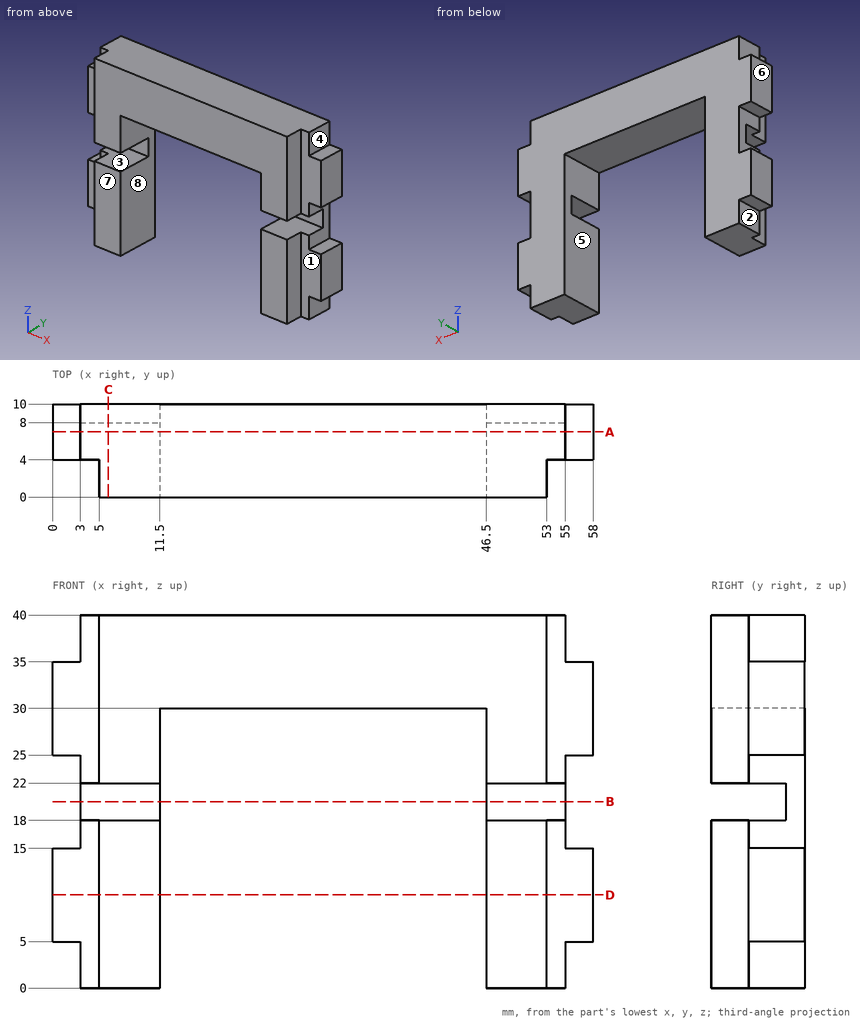
Print and shaded views of the part. All mm, measured from the part's lowest x, y and z. A direction names the side the tool comes from. Round coordinates to 2 decimals unless told otherwise and drop trailing zeros. Loops run counter-clockwise (first coordinate to the right, second up) from the corner with the lowest first, then second, coordinate; pieces in that order, holes last. Notation, with made-up numbers: M 68,1.25 L 120,1.25 A6 cw 120,11.25 Z; hole C 28,74.5 d2. An arc over 180 degrees is marked long. One line per question, with ' | ' between items.
1) Band-saw the part on C-C (x = 6). Give the cut face in (y, z), then the cut area to 3 significant figures.
Solved:
outline: M 0,0 L 10,0 L 10,40 L 0,40 L 0,22 L 8,22 L 8,18 L 0,18 Z | area: 368 mm²
2) Band-saw the part on D-D (z = 10). Give the cut face in (x, y), then the cut area to 3 significant figures.
Solved:
outline: M 0,4 L 5,4 L 5,0 L 11.5,0 L 11.5,10 L 0,10 Z; M 46.5,0 L 53,0 L 53,4 L 58,4 L 58,10 L 46.5,10 Z | area: 190 mm²
3) Drill centre lines: line 1 along Z through (x, y) = (50.5, 2.75); line 2 along X through (y, z) = (8.75, 26); line 3 along X through (y, z) = (2.75, 14). Where is each one in solid material? Low to high.
Solved:
line 1: z = 0 to 18, 22 to 40 | line 2: x = 0 to 11.5, 46.5 to 58 | line 3: x = 5 to 11.5, 46.5 to 53
4) Band-saw the part on B-B (z = 20). Give the cut face in (x, y), then the cut area to 3 significant figures.
Solved:
outline: M 3,8 L 11.5,8 L 11.5,10 L 3,10 Z; M 46.5,8 L 55,8 L 55,10 L 46.5,10 Z | area: 34.0 mm²
5) 3-axis set-ups, long thin cutter, end or side, ignore diameter. For the marked faces 1, 2, 3, 4 and 5: which of +Z, -Z, +X, -X, +Y, -Y reach the whole face in a straight line?
Solved:
face 1: +Z, -Z, +X, -Y | face 2: -Z, -X, +Y, -Y | face 3: +X, -X, -Y | face 4: +Z, +X, +Y, -Y | face 5: -Z, +Y, -Y
6) Flat gauge pins, fed straight in: pin 1 (3 mm diameter, centred on x = 31, y = 2.5, fed in from -Z); pin 2 (1.5 mm diameter, centred on y = 8.5, z = 2.5, fed in from +X); pin 3 (2.5 mm diameter, centred on x = 2, y = 6, fed in from -Z); pin 4 (0.9 mm diameter, centred on x = 1, y = 7, fed in from +Z). Where does each tip first touch, or does it go through?
Solved:
pin 1: stops at z = 30 | pin 2: stops at x = 55 | pin 3: stops at z = 0 | pin 4: stops at z = 35
7) Band-saw the part on A-A (y = 7). Give the number of separate pieces and of enclosed holes in the cut face, then the cut area to 3 significant figures.
Solved:
separate pieces: 3 | enclosed holes: 0 | area: 1,080 mm²
8) Mould opens along X. For the marked faces 6, 7 and 8 say: +X half, -X half, draft (parallel to the pull), parting line (faces both ways), or undercut.
Solved:
face 6: -X half | face 7: draft | face 8: undercut
